```python
from build123d import *

# Parameters (mm, degrees)
F0_R     = 9.68375
F0_R_2   = 6.50875
F1_DEPTH = 33.02
F3_DEPTH = 25
F4_DEPTH = 54.6


with BuildPart() as f1:
    # F0 (on Top) → F1 (new body)
    with BuildSketch(Plane.XY):
        Circle(F0_R)
        Circle(F0_R_2, mode=Mode.SUBTRACT)
    extrude(amount=F1_DEPTH)

    # F2 (on Right) → F3 (cut)
    with BuildSketch(Plane.YZ):
        with BuildLine():
            ThreePointArc((7.586009, 0), (0, 7.586009), (-7.586009, 0))
            Line((-7.586009, 0), (7.586009, 0))
        make_face()
    extrude(amount=-F3_DEPTH, mode=Mode.SUBTRACT)

    # F2 (on Right) → F4 (cut)
    with BuildSketch(Plane.YZ):
        with BuildLine():
            ThreePointArc((7.586009, 0), (0, 7.586009), (-7.586009, 0))
            Line((-7.586009, 0), (7.586009, 0))
        make_face()
    extrude(amount=F4_DEPTH, mode=Mode.SUBTRACT)


solid = f1.part
```
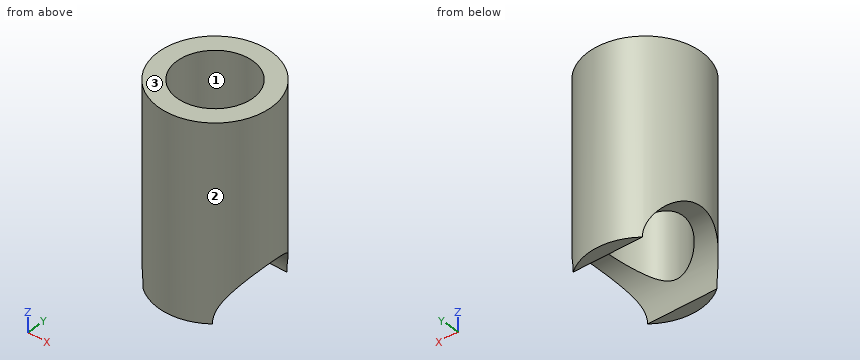
For this review, take the finished solid that the model builds, in its own axes (mm). Face numbers are marked on the shaded views. Round coordinates to 2 decimals unless told otherwise and drop trailing zeros. Order: outer loops, then holes, each group sorted by start corner. A loop starts at its lowest first (then second) coordinate and runs counter-clockwise, first axis right, second up. Notation, with made-up numbers: (5.5, 51.25) -> (11.5, 51.25) arc R23 cw to (11.5, 63.25) -> close; hole circle Ø5 at (-19, 0.5). An arc over 180 degrees is marked (long way). Use a Markdown table: item, result.
Item 1: Take a section at D-D (y = -7). State the section outline as (x, z) points.
Resolved:
| item | result |
|---|---|
| outline | (-6.69, 2.92) -> (6.69, 2.92) -> (6.69, 33.02) -> (-6.69, 33.02) -> close |
Item 2: Draft analysis for pull direction Y (two halves, no side actions). For the marked faces 1, 2 and 3, state which applies: +Y half, -Y half, draft (parallel to the pull), parting line (faces both ways), or undercut.
Resolved:
| item | result |
|---|---|
| face 1 | undercut |
| face 2 | parting line |
| face 3 | draft |
Item 3: Take a section at C-C (z = 10). State the section outline as (x, y) points, plus the area to 3 significant figures.
Resolved:
| item | result |
|---|---|
| outline | circle Ø19.37 at (0, 0); hole circle Ø13.02 at (0, 0) |
| area | 162 mm² |
Item 4: Take a section at A-A (x = 0). State the section outline as (y, z) points, plus the area to 3 significant figures.
Resolved:
| item | result |
|---|---|
| outline | (-9.68, 0) -> (-7.59, 0) arc R7.59 cw to (-6.51, 3.9) -> (-6.51, 33.02) -> (-9.68, 33.02) -> close; (6.51, 3.9) arc R7.59 cw to (7.59, 0) -> (9.68, 0) -> (9.68, 33.02) -> (6.51, 33.02) -> close |
| area | 204 mm² |
Item 5: Take a section at B-B (y = 0). State the section outline as (x, z) points, plus the area to 3 significant figures.
Resolved:
| item | result |
|---|---|
| outline | (-9.68, 7.59) -> (-6.51, 7.59) -> (-6.51, 33.02) -> (-9.68, 33.02) -> close; (6.51, 7.59) -> (9.68, 7.59) -> (9.68, 33.02) -> (6.51, 33.02) -> close |
| area | 162 mm² |
Item 6: For line 1 along X through (y, z) = (0, 26.75); line 2 along X through (y, z) = (-2, 9.5), list the stretches that pass through material, from the lowest coordinate up. Write a range as [from, to].
Resolved:
| item | result |
|---|---|
| line 1 | x = [-9.68, -6.51], [6.51, 9.68] |
| line 2 | x = [-9.47, -6.19], [6.19, 9.47] |
Item 7: For pin 1 (5 mm diameter, centred on x = -3, y = 0, fed in from -Z); pin 2 (10 mm diameter, centred on y = -5.5, z = 28, fed in from +X); pin 3 (1.5 mm diameter, centred on x = -6.5, z = 12.5, fed in from -Y); pin 4 (4 mm diameter, centred on y = -6, z = 13.5, fed in from -X), all flat-tipped, find the tip position at first contact; note any pin that passes through.
Resolved:
| item | result |
|---|---|
| pin 1 | passes through |
| pin 2 | stops at x = 9.67 |
| pin 3 | stops at y = -7.79 |
| pin 4 | stops at x = -8.82 |
